from build123d import *

# Parameters (mm, degrees)
F0_R      = 4.4
F1_DEPTH  = 69
F2_W      = 30
F2_H      = 59
F3_DEPTH  = 70.001
F4_W      = 19
F4_H      = 20
F4_R      = 4.4
F5_DEPTH  = 63
F7_DEPTH  = 70.001
F8_W      = 40
F8_H      = 39
F9_DEPTH  = 45.001
F10_R     = 4
F11_DEPTH = 69.001
F12_R     = 3
F13_DEPTH = 17.3552487891
F15_DEPTH = 69.001
F16_R     = 1.25
F17_DEPTH = 25


with BuildPart() as f1:
    # F0 (on Top) → F1 (new body)
    with BuildSketch(Plane.XY):
        Polygon((-35, -37.5), (35, -37.5), (35, 37.5), (10, 37.5), (10, 17.5), (29, 17.5), (29, -2.5), (-29, -2.5), (-29, 17.5), (-10, 17.5), (-10, 37.5), (-35, 37.5), align=None)
        with Locations((-20, 27.5)):
            Circle(F0_R, mode=Mode.SUBTRACT)
        with Locations((20, 27.5)):
            Circle(F0_R, mode=Mode.SUBTRACT)
    extrude(amount=F1_DEPTH)

    # F2 (on face) → F3 (cut, through all)
    with BuildSketch(Plane(origin=(-35, 0, 0), x_dir=(0, -1, 0), z_dir=(-1, 0, 0))):
        with Locations((22.5, 29.5)):
            Rectangle(F2_W, F2_H)
    extrude(amount=-F3_DEPTH, mode=Mode.SUBTRACT)

    # F4 (on face) → F5 (cut)
    with BuildSketch(Plane.XY.offset(69)):
        with Locations((19.5, 27.5)):
            Rectangle(F4_W, F4_H)
        with Locations((20, 27.5)):
            Circle(F4_R, mode=Mode.SUBTRACT)
        with Locations((-19.5, 27.5)):
            Rectangle(F4_W, F4_H)
        with Locations((-20, 27.5)):
            Circle(F4_R, mode=Mode.SUBTRACT)
    extrude(amount=-F5_DEPTH, mode=Mode.SUBTRACT)

    # F6 (on face) → F7 (cut, through all)
    with BuildSketch(Plane(origin=(-35, 0, 0), x_dir=(0, -1, 0), z_dir=(-1, 0, 0))):
        Polygon((2.5, 69), (-37.5, 69), (-37.5, 6), align=None)
    extrude(amount=-F7_DEPTH, mode=Mode.SUBTRACT)

    # F8 (on face) → F9 (cut, through all)
    with BuildSketch(Plane.XZ.offset(7.5)):
        with Locations((0, 39.5)):
            Rectangle(F8_W, F8_H)
    extrude(amount=-F9_DEPTH, mode=Mode.SUBTRACT)

    # F10 (on face) → F11 (cut, through all)
    with BuildSketch(Plane.XY.offset(69)):
        with Locations((0, -17.5)):
            Circle(F10_R)
    extrude(amount=-F11_DEPTH, mode=Mode.SUBTRACT)

    # F12 (on face) → F13 (cut, through all)
    with BuildSketch(Plane.XZ.offset(37.5)):
        with Locations((0, 64)):
            Circle(F12_R)
    extrude(amount=-F13_DEPTH, mode=Mode.SUBTRACT)

    # F14 (on face) → F15 (cut, through all)
    with BuildSketch(Plane.XY.offset(69)):
        Polygon((-15, -7.5), (-35, -7.5), (-35, -37.5), (-6, -37.5), align=None)
        Polygon((15, -7.5), (6, -37.5), (35, -37.5), (35, -7.5), align=None)
    extrude(amount=-F15_DEPTH, mode=Mode.SUBTRACT)

    # F16 (on face) → F17 (cut)
    with BuildSketch(Plane.XZ.offset(7.5)):
        with Locations((-32, 50)):
            Circle(F16_R)
        with Locations((-32, 10)):
            Circle(F16_R)
        with Locations((32, 50)):
            Circle(F16_R)
        with Locations((32, 10)):
            Circle(F16_R)
    extrude(amount=-F17_DEPTH, mode=Mode.SUBTRACT)


solid = f1.part
Geometry check sheet. Reference: the model listing, model coordinates, mm. A direction names the side the tool comes from. Give positions to 0.01 mm unless a question says otherwise; leave off trailing zeros. Order: outer loops, then holes, each group sorted by start corner. A loop starts at its lowest first (then second) coordinate and runs counter-clockwise, first axis right, second up. Notation, with made-up numbers: (-32, 46) - (-16, 46) arc R12 ccw to (-16, 53) - close; hole circle Ø4 at (13, 23.5). An arc over 180 degrees is marked (long way). Answer as a JSON object with one key per item and string values.
(1) Cross-section at B-B (y = -17.5). Record the cut outline in (x, z).
Report:
{"outline": "(-12, 59) - (-4, 59) - (-4, 69) - (-12, 69) - close; (4, 59) - (12, 59) - (12, 69) - (4, 69) - close"}
(2) Cross-section at C-C (x = 13.5). Record the cut outline in (y, z).
Report:
{"outline": "(-12.5, 59) - (-2.5, 59) - (-2.5, 69) - (-12.5, 69) - close; (-7.5, 0) - (-2.5, 0) - (-2.5, 20) - (-7.5, 20) - close; (17.5, 0) - (37.5, 0) - (37.5, 6) - (17.5, 6) - close"}
(3) Depth check by flat-ended pin: pin 1 Ø11.5 at (x, y) = (-20, 27.5) entering from -Z; pin 2 Ø12 at (x, z) = (18, 30) entering from +Y; pin 3 Ø7 at (x, y) = (20, 27.5) entering from +Z; pin 4 Ø1.5 at (x, z) = (32, 10) entering from +Y. Enter the tip coordinate at first touch or a pass-through.
Report:
{"pin 1": "z = 0", "pin 2": "y = -2.5", "pin 3": "through", "pin 4": "y = 35.44"}
(4) Cross-section at A-A (x = 0). Record the cut outline in (y, z), then the cut area to 3 significant figures.
Report:
{"outline": "(-37.5, 59) - (-21.5, 59) - (-21.5, 61) - (-37.5, 61) - close; (-37.5, 67) - (-21.5, 67) - (-21.5, 69) - (-37.5, 69) - close; (-13.5, 59) - (-2.5, 59) - (-2.5, 69) - (-13.5, 69) - close; (-7.5, 0) - (-2.5, 0) - (-2.5, 20) - (-7.5, 20) - close", "area": "274 mm^2"}
(5) Cross-section at D-D (y = -29). Record the cut outline in (x, z).
Report:
{"outline": "(-8.55, 59) - (8.55, 59) - (8.55, 69) - (-8.55, 69) - close; hole circle Ø6 at (0, 64)"}
(6) Draft check along X on faces 1 (the flat face through (29, 9, 26)), 2 (the flat face through (-10.437, -22.71, 64.07)), 3 (the flat face through (10.563, -22.29, 64.07)). Enter one of: released by +X, released by -X, zero draft, split by the parting line, or undercut.
Report:
{"face 1": "undercut", "face 2": "released by -X", "face 3": "released by +X"}
(7) Material ranges on line 1 (X direction, y = 0, z = 50); line 2 (Y direction, x = 20, z = 3.4); line 3 (X direction, y = 2.5, z = 12), recorded low to high.
Report:
{"line 1": "-35 to -33.25, -30.75 to -29, 29 to 30.75, 33.25 to 35", "line 2": "-7.5 to -2.5, 17.5 to 23.1, 31.9 to 37.5", "line 3": "-35 to -29, 29 to 35"}
(8) Tool access check on faces 4 (the flat face through (-29, 8, 27)), 5 (the flat face through (20, -5, 39)), 6 (the flat face through (19, 17.5, 3)), 7 (the flat face through (32, 17.5, 10)), 8 (the flat face through (-10, 27, 3)). Record the directions out of +Z, -Z, +X, -X, +Y, -Y that give a thin tool (end or side, any length) a straight path to the whole face; none if there is none.
Report:
{"face 4": "+Z", "face 5": "+Y, -Y", "face 6": "+Z, -Z", "face 7": "-Y", "face 8": "+Z, -Z, +Y"}
